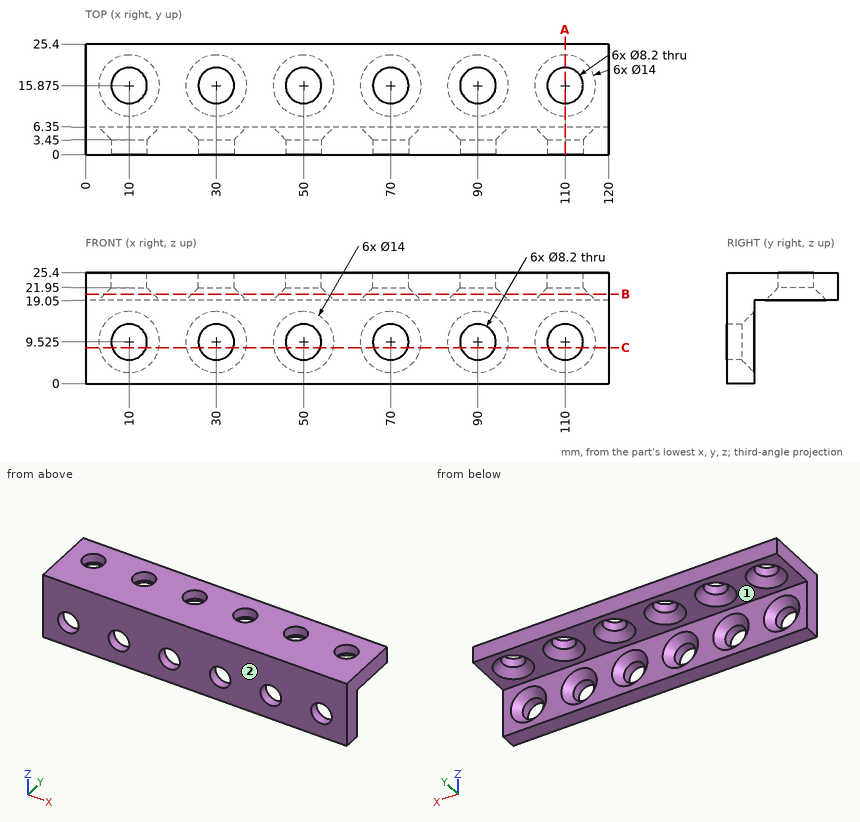
Input: dimensioned drawing with shaded views. Units: mm. Origin: part minimum x, y, z. A direction names the side the tool comes from. Coordinates: 2 decimals unless noted, no trailing zeros. Loops run counter-clockwise (first coordinate to the right, second up) from the corner with the lowest first, then second, coordinate; pieces in that order, holes last. Notation, with made-up numbers: M 43.5,68.5 L 53.5,68.5 A11 cw 53.5,80.5 Z; hole C 74,88 d9. An arc over 180 degrees is marked long. One line per item, written item: value. Start each with the question number.
1) Material intervals for L1, parallel to Y at x = 90, z = 22.95 (3 decimals); L2, parallel to Z at x = 110, y = 2.5 (3 decimals); L3, parallel to Z at x = 16, y = 11, sorted ascending. Write a range as from..to.
2) Pin query (flat end, axial travel): P1, Ø9.5, axis at x = 43, z = 7, coming from the +Y side; P2, Ø6.5, axis at x = 90, z = 9.525, coming from the +Y side; P3, Ø8, axis at x = 90.5, z = 11.5, coming from the +Y side. Return the tip coordinate at first contact, or that it passes through.
3) Cut plane B-B (z = 20.5). Return loops of the section in (x, y) (3 decimals).
4) Reachability of the marked faces 1 and 2 from +Z, -Z, +X, -X, +Y, -Y: full face, straight path, thin tool, end or side. Return the list, or none.
5) Cut plane C-C (z = 8.25). Count the separate pieces of the cut face and the enclosed holes in it, then the cut area to 3 significant figures.
6) Cut plane A-A (x = 110). Return loops of the section in (y, z) (3 decimals), then the cut area to 3 significant figures.
Evaluation:
1. L1: 0..11.775, 19.975..25.4
1. L2: 0..5.425, 13.625..25.4
1. L3: 19.05..25.4
2. P1: y = 6.35
2. P2: through
2. P3: y = 5.39
3. outline: M 0,0 L 120,0 L 120,25.4 L 0,25.4 Z; hole C 10,15.875 d11.1; hole C 30,15.875 d11.1; hole C 50,15.875 d11.1; hole C 70,15.875 d11.1; hole C 90,15.875 d11.1; hole C 110,15.875 d11.1
4. face 1: -Z, +X, -X, +Y
4. face 2: +Z, -Z, +X, -X, -Y
5. separate pieces: 7
5. enclosed holes: 0
5. area: 413 mm^2
6. outline: M 0,0 L 6.35,0 L 6.35,2.525 L 3.45,5.425 L 0,5.425 Z; M 0,13.625 L 3.45,13.625 L 6.35,16.525 L 6.35,19.05 L 8.875,19.05 L 11.775,21.95 L 11.775,25.4 L 0,25.4 Z; M 19.975,21.95 L 22.875,19.05 L 25.4,19.05 L 25.4,25.4 L 19.975,25.4 Z
6. area: 161 mm^2
